Verification items for the finished model (mm, model axes). Face numbers are marked on the shaded views. A direction names the side the tool comes from. Coordinates: 2 decimals unless noted, no trailing zeros. Loops run counter-clockwise (first coordinate to the right, second up) from the corner with the lowest first, then second, coordinate; pieces in that order, holes last. Notation, with made-up numbers: (33, 61.25) - (85, 61.25) arc R12 cw to (85, 77.25) - close; hole circle Ø10 at (32, -11.75). An arc over 180 degrees is marked (long way). Answer as CSV lines item,"result". Start each with the question number.
1. Cross-section at A-A (z = 7.95). Enter the section's corners in (x, y).
2. Material ranges on line 1 (Y direction, x = 91, z = 46.5); line 2 (X direction, y = -3.25, z = 21.5); line 3 (Z direction, x = 45, y = -13.5), recorded low to high. Write a range as [from, to].
3. Cross-section at D-D (y = -8.25). Enter the section's corners in (x, z).
4. Cross-section at C-C (x = 62.5). Enter the section's corners in (y, z), plus the area to 3 significant figures.
5. Cross-section at B-B (z = 21). Enter the section's corners in (x, y).
6. Set-up check for the marked faces 1, 2 and 3: record each of +Z, -Z, +X, -X, +Y, -Y from which the full face is reachable in a straight line by a thin tool's end or side.
7. Gauge pin test, flat ends, axial feed: P1, Ø4.5, axis at x = 7.18, z = 7.95, coming from the +Y side; P2, Ø2.5, axis at x = 34.5, y = -11.5, coming from the +Z side; P3, Ø3.5, axis at x = 92.91, z = 62.05, coming from the +Y side; P4, Ø4.5, axis at x = 57.5, y = -5.5, coming from the +Z side. Record the tip position at first contact, or that the pin passes through.
```python
from build123d import *

# Parameters (mm, degrees)
F0_R     = 2
F0_W     = 80.502108
F0_H     = 36.524102
F1_DEPTH = 1
F0_W_2   = 70.236466
F0_H_2   = 22.275392
F2_DEPTH = 10
F3_DEPTH = 15


with BuildPart() as f1:
    # F0 (on Front) → F1 (new body)
    with BuildSketch(Plane.XZ):
        with BuildLine():
            ThreePointArc((4.3625, 70), (3.084753, 66.915247), (0, 65.6375))
            Line((0, 65.6375), (0, 4.3625))
            ThreePointArc((0, 4.3625), (3.084753, 3.084753), (4.3625, 0))
            Line((4.3625, 0), (95.728963, 0))
            ThreePointArc((95.728963, 0), (97.00671, 3.084753), (100.091463, 4.3625))
            Line((100.091463, 4.3625), (100.091463, 65.6375))
            ThreePointArc((100.091463, 65.6375), (97.00671, 66.915247), (95.728963, 70))
            Line((95.728963, 70), (4.3625, 70))
        make_face()
        with Locations((7.183232, 7.95)):
            Circle(F0_R, mode=Mode.SUBTRACT)
        with Locations((47, 34)):
            Rectangle(F0_W, F0_H, mode=Mode.SUBTRACT)
        with Locations((92.908232, 7.95)):
            Circle(F0_R, mode=Mode.SUBTRACT)
        with Locations((7.183232, 62.05)):
            Circle(F0_R, mode=Mode.SUBTRACT)
        with Locations((92.908232, 62.05)):
            Circle(F0_R, mode=Mode.SUBTRACT)
    extrude(amount=F1_DEPTH)

    # F0 (on Front) → F2 (join)
    with BuildSketch(Plane.XZ):
        with Locations((47, 34)):
            Rectangle(F0_W, F0_H)
        with Locations((47, 34)):
            Rectangle(F0_W_2, F0_H_2, mode=Mode.SUBTRACT)
    extrude(amount=F2_DEPTH)

    # F0 (on Front) → F3 (join)
    with BuildSketch(Plane.XZ):
        with Locations((47, 34)):
            Rectangle(F0_W_2, F0_H_2)
    extrude(amount=F3_DEPTH)


solid = f1.part
```
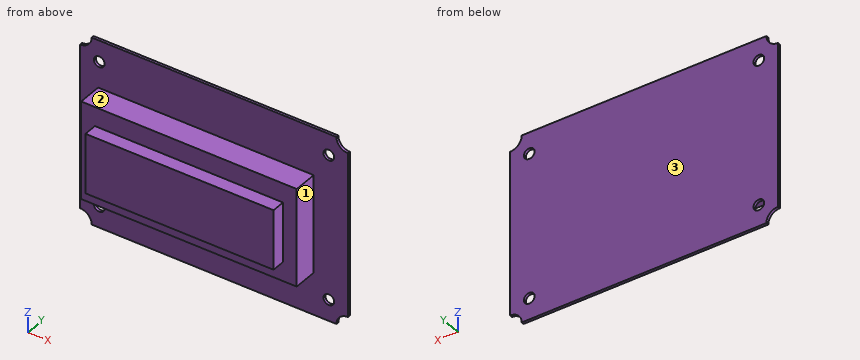
Values follow:
1,outline,"(0, -1) - (5.18, -1) - (5.18, 0) - (0, 0) - close; (9.18, -1) - (90.91, -1) - (90.91, 0) - (9.18, 0) - close; (94.91, -1) - (100.09, -1) - (100.09, 0) - (94.91, 0) - close"
2,line 1,"y = [-1, 0]"
2,line 2,"x = [6.75, 87.25]"
2,line 3,"z = [22.86, 45.14]"
3,outline,"(6.75, 15.74) - (87.25, 15.74) - (87.25, 52.26) - (6.75, 52.26) - close"
4,outline,"(-15, 22.86) - (-10, 22.86) - (-10, 15.74) - (-1, 15.74) - (-1, 0) - (0, 0) - (0, 70) - (-1, 70) - (-1, 52.26) - (-10, 52.26) - (-10, 45.14) - (-15, 45.14) - close"
4,area,"510 mm²"
5,outline,"(0, -1) - (6.75, -1) - (6.75, -10) - (87.25, -10) - (87.25, -1) - (100.09, -1) - (100.09, 0) - (0, 0) - close"
6,face 1,"+Z, -Z, +X, -Y"
6,face 2,"+Z, +X, -X, -Y"
6,face 3,"+Z, -Z, +X, -X, +Y"
7,P1,"stops at y = 0"
7,P2,"stops at z = 45.14"
7,P3,"passes through"
7,P4,"stops at z = 52.26"
